from build123d import *

# Parameters (mm, degrees)
F0_R     = 19.05
F0_R_2   = 3.175
F1_DEPTH = 3.81
F3_DEPTH = 3.7338
F5_DEPTH = 6.35
F6_DEPTH = 10.1092


with BuildPart() as f1:
    # F0 (on Front) → F1 (new body)
    with BuildSketch(Plane.XZ):
        Circle(F0_R)
        Circle(F0_R_2, mode=Mode.SUBTRACT)
    extrude(amount=F1_DEPTH)

    # F2 (on Front) → F3, piece 2 (join)
    with BuildSketch(Plane.XZ):
        with BuildLine():
            Line((19.3002153026, -14.8442822065), (15.2105484158, -9.9704070017))
            Line((15.2105484158, -9.9704070017), (11.9190644701, -13.8930448189))
            Line((11.9190644701, -13.8930448189), (17.4290577612, -17.0742409287))
            ThreePointArc((17.4290577612, -17.0742409287), (18.2845909468, -17.2250945122), (19.036934204, -16.7907289302))
            Line((19.036934204, -16.7907289302), (19.3002153026, -16.4769627351))
            ThreePointArc((19.3002153026, -16.4769627351), (19.5973388598, -15.6606224708), (19.3002153026, -14.8442822065))
        make_face()
        with BuildLine():
            Line((11.9828917218, -21.0592770188), (10.1196430624, -14.9758290499))
            Line((10.1196430624, -14.9758290499), (5.5582912351, -17.3028493588))
            Line((5.5582912351, -17.3028493588), (9.3898339973, -22.3821519505))
            ThreePointArc((9.3898339973, -22.3821519505), (10.1186515435, -22.8549297204), (10.9808538675, -22.7486236155))
            Line((10.9808538675, -22.7486236155), (11.3457098838, -22.5624885854))
            ThreePointArc((11.3457098838, -22.5624885854), (11.9378629358, -21.9268404135), (11.9828917218, -21.0592770188))
        make_face()
        with BuildLine():
            Line((3.3225191024, -24.1014032107), (3.9599463344, -17.7710223943))
            Line((3.9599463344, -17.7710223943), (-1.1466123432, -18.1505121598))
            Line((-1.1466123432, -18.1505121598), (0.4195197448, -24.3171372529))
            ThreePointArc((0.4195197448, -24.3171372529), (0.9084468903, -25.0352208705), (1.7445620653, -25.2710285242))
            Line((1.7445620653, -25.2710285242), (2.1530283986, -25.24067368))
            ThreePointArc((2.1530283986, -25.24067368), (2.9451040203, -24.8838683481), (3.3225191024, -24.1014032107))
        make_face()
        with BuildLine():
            Line((-6.024496716, -23.4720864394), (-3.1015451532, -17.8208574653))
            Line((-3.1015451532, -17.8208574653), (-7.9892249639, -16.2939193272))
            Line((-7.9892249639, -16.2939193272), (-8.8030668347, -22.604045805))
            ThreePointArc((-8.8030668347, -22.604045805), (-8.6128057983, -23.4516863972), (-7.9222045185, -23.9787193257))
            Line((-7.9222045185, -23.9787193257), (-7.531245993, -24.100856926))
            ThreePointArc((-7.531245993, -24.100856926), (-6.6634444839, -24.0606776264), (-6.024496716, -23.4720864394))
        make_face()
        with BuildLine():
            Line((-14.6087634205, -19.377536382), (-9.5885228366, -15.4689280316))
            Line((-9.5885228366, -15.4689280316), (-13.3881088706, -12.0361303417))
            Line((-13.3881088706, -12.0361303417), (-16.7687691136, -17.4260441702))
            ThreePointArc((-16.7687691136, -17.4260441702), (-16.9508230748, -18.275485275), (-16.5442742828, -19.0432169437))
            Line((-16.5442742828, -19.0432169437), (-16.2403508241, -19.3178015268))
            ThreePointArc((-16.2403508241, -19.3178015268), (-15.4354279769, -19.6445935792), (-14.6087634205, -19.377536382))
        make_face()
        with BuildLine():
            Line((-20.5652638633, -12.7449498911), (-14.5090268925, -10.7950707898))
            Line((-14.5090268925, -10.7950707898), (-16.9009077473, -6.2673936827))
            Line((-16.9009077473, -6.2673936827), (-21.9250110088, -10.1710357224))
            ThreePointArc((-21.9250110088, -10.1710357224), (-22.3873392768, -10.9065263124), (-22.2687390391, -11.7671236741))
            Line((-22.2687390391, -11.7671236741), (-22.0774159066, -12.1292860977))
            ThreePointArc((-22.0774159066, -12.1292860977), (-21.4333815325, -12.7123071611), (-20.5652638633, -12.7449498911))
        make_face()
        with BuildLine():
            Line((-23.8361925967, -4.2197788404), (-17.4791440368, -4.48048627))
            Line((-17.4791440368, -4.48048627), (-18.1609497484, 0.5945600333))
            Line((-18.1609497484, 0.5945600333), (-24.2237885625, -1.3346937785))
            ThreePointArc((-24.2237885625, -1.3346937785), (-24.9115978854, -1.8653652124), (-25.0973813726, -2.713998426))
            Line((-25.0973813726, -2.713998426), (-25.0428447078, -3.1199441296))
            ThreePointArc((-25.0428447078, -3.1199441296), (-24.6396722009, -3.8894542108), (-23.8361925967, -4.2197788404))
        make_face()
        with BuildLine():
            Line((-23.5361590974, 5.4379167113), (-17.8682561964, 2.5474303402))
            Line((-17.8682561964, 2.5474303402), (-16.3693803408, 7.4437886991))
            Line((-16.3693803408, 7.4437886991), (-22.6840714351, 8.2214204499))
            ThreePointArc((-22.6840714351, 8.2214204499), (-23.5306066884, 8.0263002296), (-24.053669455, 7.3326870971))
            Line((-24.053669455, 7.3326870971), (-24.1735623934, 6.9410343869))
            ThreePointArc((-24.1735623934, 6.9410343869), (-24.1284057917, 6.0734776356), (-23.5361590974, 5.4379167113))
        make_face()
        with BuildLine():
            Line((-19.5623090328, 14.1900364797), (-15.4726421461, 9.3161612749))
            Line((-15.4726421461, 9.3161612749), (-12.1811582004, 13.2387990921))
            Line((-12.1811582004, 13.2387990921), (-17.6911514915, 16.419995202))
            ThreePointArc((-17.6911514915, 16.419995202), (-18.5466846771, 16.5708487855), (-19.2990279342, 16.1364832035))
            Line((-19.2990279342, 16.1364832035), (-19.5623090328, 15.8227170083))
            ThreePointArc((-19.5623090328, 15.8227170083), (-19.8594325901, 15.006376744), (-19.5623090328, 14.1900364797))
        make_face()
        with BuildLine():
            Line((-12.2220281822, 20.5830006913), (-10.324199684, 14.5102515817))
            Line((-10.324199684, 14.5102515817), (-5.7761605757, 16.8631847042))
            Line((-5.7761605757, 16.8631847042), (-9.6365385319, 21.9206066554))
            ThreePointArc((-9.6365385319, 21.9206066554), (-10.3680340136, 22.3892303804), (-11.2296175865, 22.2780207486))
            Line((-11.2296175865, 22.2780207486), (-11.5934087375, 22.0898129895))
            ThreePointArc((-11.5934087375, 22.0898129895), (-12.1819358724, 21.4508062237), (-12.2220281822, 20.5830006913))
        make_face()
        with BuildLine():
            Line((-3.0776811638, 23.6942735067), (-3.6322001833, 17.3560921103))
            Line((-3.6322001833, 17.3560921103), (1.4689542355, 17.8023852928))
            Line((1.4689542355, 17.8023852928), (-0.1777540434, 23.9479842548))
            ThreePointArc((-0.1777540434, 23.9479842548), (-0.6760377686, 24.6596071637), (-1.5151676361, 24.8844513341))
            Line((-1.5151676361, 24.8844513341), (-1.9232016905, 24.84875298))
            ThreePointArc((-1.9232016905, 24.84875298), (-2.7105395093, 24.4816113255), (-3.0776811638, 23.6942735067))
        make_face()
        with BuildLine():
            Line((6.9191977973, 23.0382329287), (3.7380016875, 17.5282396376))
            Line((3.7380016875, 17.5282396376), (8.5498293092, 15.7768776109))
            Line((8.5498293092, 15.7768776109), (9.6546471237, 22.0426107965))
            ThreePointArc((9.6546471237, 22.0426107965), (9.5037935402, 22.8981439822), (8.8383068594, 23.4565536106))
            Line((8.8383068594, 23.4565536106), (8.4534156421, 23.5966425571))
            ThreePointArc((8.4534156421, 23.5966425571), (7.5846844781, 23.5966425571), (6.9191977973, 23.0382329287))
        make_face()
        with BuildLine():
            Line((15.9169355088, 18.1412522665), (10.5493562296, 14.7252418101))
            Line((10.5493562296, 14.7252418101), (14.0070511629, 10.9482986337))
            Line((14.0070511629, 10.9482986337), (17.8825814171, 15.9941186865))
            ThreePointArc((17.8825814171, 15.9941186865), (18.1441998983, 16.8225205248), (17.8121248444, 17.6252782679))
            Line((17.8121248444, 17.6252782679), (17.5355487664, 17.9273905568))
            ThreePointArc((17.5355487664, 17.9273905568), (16.7651617859, 18.328884935), (15.9169355088, 18.1412522665))
        make_face()
        with BuildLine():
            Line((21.2552525466, 11.001283816), (15.1096535847, 9.3545755371))
            Line((15.1096535847, 9.3545755371), (17.2737295605, 4.7136996305))
            Line((17.2737295605, 4.7136996305), (22.4854961538, 8.3630178866))
            ThreePointArc((22.4854961538, 8.3630178866), (22.983779879, 9.0746407955), (22.9080649691, 9.9400661752))
            Line((22.9080649691, 9.9400661752), (22.7349636234, 10.311283209))
            ThreePointArc((22.7349636234, 10.311283209), (22.1206779263, 10.9255689062), (21.2552525466, 11.001283816))
        make_face()
        with BuildLine():
            Line((23.9182224306, 1.9714912908), (17.6524892449, 3.0763091054))
            Line((17.6524892449, 3.0763091054), (17.6524892449, -2.0443308946))
            Line((17.6524892449, -2.0443308946), (23.9182224306, -0.9395130801))
            ThreePointArc((23.9182224306, -0.9395130801), (24.6705656877, -0.505147498), (24.9676892449, 0.3111927663))
            Line((24.9676892449, 0.3111927663), (24.9676892449, 0.7207854445))
            ThreePointArc((24.9676892449, 0.7207854445), (24.6705656877, 1.5371257088), (23.9182224306, 1.9714912908))
        make_face()
        with BuildLine():
            Line((23.229211427, -6.6084690539), (17.6019985229, -3.6395450588))
            Line((17.6019985229, -3.6395450588), (16.0352661171, -8.5146146561))
            Line((16.0352661171, -8.5146146561), (22.338548369, -9.379870462))
            ThreePointArc((22.338548369, -9.379870462), (23.1877118276, -9.196525825), (23.7203571155, -8.5102439349))
            Line((23.7203571155, -8.5102439349), (23.8456778024, -8.1202940823))
            ThreePointArc((23.8456778024, -8.1202940823), (23.8125742696, -7.2521938626), (23.229211427, -6.6084690539))
        make_face()
    extrude(amount=F3_DEPTH)

    # F5 (add): a face of the model
    f5_faces = [f1.faces().sort_by_distance(p)[0] for p in [
        (-18.5111846327, -3.81, 0),
    ]]
    extrude(f5_faces, amount=F5_DEPTH)

    # F6 (add): a face of the model
    f6_faces = [f1.faces().sort_by_distance(p)[0] for p in [
        (24.1275892459, 0, -0.049536166),
    ]]
    extrude(f6_faces, amount=-F6_DEPTH)


with BuildPart() as f3:
    # F2 (on Front) → F3 (new body)
    with BuildSketch(Plane.XZ):
        with BuildLine():
            Line((-44.3880631869, 14.6072879799), (-45.4928810014, 8.3415547942))
            Line((-45.4928810014, 8.3415547942), (-40.3722410014, 8.3415547942))
            Line((-40.3722410014, 8.3415547942), (-41.477058816, 14.6072879799))
            ThreePointArc((-41.477058816, 14.6072879799), (-41.911424398, 15.359631237), (-42.7277646623, 15.6567547942))
            Line((-42.7277646623, 15.6567547942), (-43.1373573405, 15.6567547942))
            ThreePointArc((-43.1373573405, 15.6567547942), (-43.9536976048, 15.359631237), (-44.3880631869, 14.6072879799))
        make_face()
    extrude(amount=F3_DEPTH)


solid = f1.part
Can you work these out from the model? Positions are in its coordinate system, mm. A direction names the side the tool comes from. Round coordinates to 2 decimals unless told otherwise and drop trailing zeros. Order: outer loops, then holes, each group sorted by start corner. A loop starts at its lowest first (then second) coordinate and runs counter-clockwise, first axis right, second up. Notation, with made-up numbers: M 86.25,9 L 115.25,9 A27 ccw 115.25,39 Z; hole C 43.5,-21 d10. An arc over 180 degrees is marked long. Use a Markdown table: item, result.
1) Imagine slicing it at B-B (z = -6). List the corners of the cut face in (x, y) for me.
Geometry says:
| item | result |
|---|---|
| outline | M -18.08,-10.16 L 18.08,-10.16 L 18.08,-10.11 L 22.08,-10.11 L 22.08,0 L -18.08,0 Z |
2) If we mould it in two halves opening along X, with no side actions, what happens to faces 6 (the face through (-21.44, -4.98, -12.71)), 7 (the face through (-12.18, -4.98, 21.46)), 8 (the face through (15, -10.109, 15))? For each: +X half, -X half, draft (parallel to the pull), parting line (faces both ways), or undercut.
Geometry says:
| item | result |
|---|---|
| face 6 | undercut |
| face 7 | -X half |
| face 8 | draft |
3) I'm going to push flat-ended pins straight in: P1, Ø2.5, axis at x = 6.5, z = 20, coming from the -Y side; P2, Ø2, axis at y = -1.5, z = -3.5, coming from the +X side; P3, Ø5, axis at x = 0, z = 0, coming from the -Y side (3 decimals); P4, Ø1, axis at y = -3.5, z = -12.5, coming from the +X side. Where does each tip first touch, or does it pass through?
Geometry says:
| item | result |
|---|---|
| P1 | stops at y = -10.11 |
| P2 | stops at x = 19.23 |
| P3 | passes through |
| P4 | stops at x = 17.75 |
4) If I drill on line 1 along Z through (x, y) = (20.5, -1.5); line 2 along X through (y, z) = (-6.5, -18); line 3 along Y through (x, z) = (16.5, 18), over which ranges is the centre line in solid material (lowest first)?
Geometry says:
| item | result |
|---|---|
| line 1 | z = -9.13 to -5.17, -1.54 to 2.57, 6.97 to 10.8 |
| line 2 | x = -16.96 to -12.84, -8.21 to 11.05 |
| line 3 | y = -10.11 to 0 |
5) On a 3-axis mill with a long thin cutter (end or side, diameter ignored), from which of +Z, -Z, +X, -X, +Y, -Y can I reach the whole of each face in a straight line? I mean faces 1 (the face through (-7, -10.109, -21)), 2 (the face through (0.49, -4.98, 21.45)), 3 (the face through (16.32, -4.98, 13.96)), 4 (the face through (20, -10.109, -7)), 5 (the face through (-4.811, -4.984, -21.126)). Say none if no direction works.
Geometry says:
| item | result |
|---|---|
| face 1 | -Z, -X, -Y |
| face 2 | +Z, +Y, -Y |
| face 3 | +X, +Y, -Y |
| face 4 | -Z, +X, -Y |
| face 5 | -Z, +Y, -Y |
6) Imagine slicing it at A-A (z = 9). List the corners of the cut face in (x, y) for me, then the cut area to 3 significant figures.
Geometry says:
| item | result |
|---|---|
| outline | M -16.79,-10.16 L 16.79,-10.16 L 16.79,-10.11 L 22.96,-10.11 L 22.96,0 L -16.79,0 Z |
| area | 404 mm² |
